from build123d import *

# Parameters (mm, degrees)
SKETCH4_W = 10.28192
SKETCH4_H = 1.12


with BuildPart() as part:
    # Sweep1: sweep along a path in Sketch1
    with BuildLine(Plane.XY) as sweep1_path:
        Line((-2.41e-07, 9.261094), (132.90351643, 9.461083519))
        ThreePointArc((132.90351643, 9.461083519), (142.178535768, 0.213935094), (132.931386612, -9.061083513))
        Line((132.931386612, -9.061083513), (0.027869908, -9.261052065))
        ThreePointArc((0.027869908, -9.261052065), (-9.247137468, -0.013914106), (-2.41e-07, 9.261094))
    # Sketch4 → Sweep1 (sweep)
    with BuildSketch(Plane.ZY):
        with Locations((5.14096, 9.821094)):
            Rectangle(SKETCH4_W, SKETCH4_H)
    sweep(path=sweep1_path.line)


solid = part.part
Build history of the part. All positions in model axes, mm. A direction names the side the tool comes from. Coordinates: 2 decimals unless noted, no trailing zeros. Write each loop counter-clockwise with the first axis right and the second up, starting at its lowest first coordinate (ties: lowest second). Pieces come first, ordered by that corner, then holes.
(1) Cut at C-C on x = 49.5. List the corners of the cut face in (y, z), and give its area (3 significant figures).
(2) Cut at B-B on z = 1.75. List the corners of the cut face in (x, y).
(3) 3-axis set-ups, long thin cutter, end or side, ignore diameter. For faces 1 (the flat face through (67, 10, 0)), 2 (the cylindrical face through (-9.245, -0.218, 5.213)): which of +Z, -Z, +X, -X, +Y, -Y reach the whole face in a straight line?
(4) Drill centre lines: line 1 (Y direction, x = 51, z = 2.5); line 2 (Y direction, x = 113.5, z = 2); line 3 (X direction, y = 3, z = 6.75). Where is each one in solid material? Low to high.
(5) Mould opens along X. For faces 3 (the cylindrical face through (142.176, 0.418, 5.213)), 4 (the flat face through (61, -10, 10.282)) say: pulls with the +X half, pulls with the -X half, needs draft (parallel to the pull), parting line crosses it, or undercut.
(6) Pin check, flat tips, straight feed: pin 1 Ø3 at (x, z) = (40, 7) entering from +Y; pin 2 Ø5 at (x, z) = (103.5, 3.5) entering from +Y; pin 3 Ø1.5 at (y, z) = (5, 1) entering from -X. Stop position of each tip, or through.
(7) Cut at A-A on y = -5.5. List the corners of the cut face in (x, z).
Working result:
1. outline: (-10.31, 0) - (-9.19, 0) - (-9.19, 10.28) - (-10.31, 10.28) - close; (9.34, 0) - (10.46, 0) - (10.46, 10.28) - (9.34, 10.28) - close
1. area: 23.0 mm2
2. outline: (0, 10.38) arc R10.38 ccw to (0.03, -10.38) - (132.93, -10.18) arc R10.38 ccw to (132.9, 10.58) - close; hole (0, 9.26) arc R9.26 ccw to (0.03, -9.26) - (132.93, -9.06) arc R9.26 ccw to (132.9, 9.46) - close
3. face 1: -Z, +X, -X, +Y, -Y
3. face 2: +Z, -Z
4. line 1: y = -10.3 to -9.18, 9.34 to 10.46
4. line 2: y = -10.21 to -9.09, 9.43 to 10.55
4. line 3: x = -9.92 to -8.75, 141.75 to 142.91
5. face 3: undercut
5. face 4: needs draft
6. pin 1: stops at y = 10.44
6. pin 2: stops at y = 10.54
6. pin 3: stops at x = -9.46
7. outline: (-8.79, 0) - (-7.44, 0) - (-7.44, 10.28) - (-8.79, 10.28) - close; (140.22, 0) - (141.59, 0) - (141.59, 10.28) - (140.22, 10.28) - close
